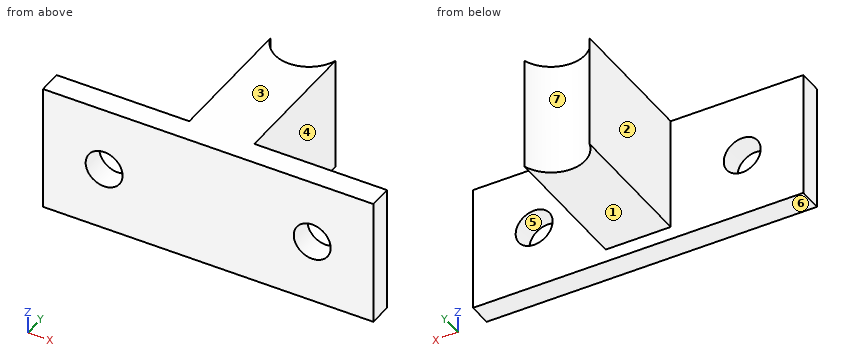
Autodesk Fusion 360 part; units mm, degrees
sketch "Sketch1" plane through (0, 0, 0) normal (0, 1, 0) x (1, 0, 0)
  line L0 (2.5, -4.375) -> (-2.5, -4.375)
  line L1 (-2.5, -4.375) -> (-2.5, 4.375)
  line L2 (-2.5, 4.375) -> (2.5, 4.375)
  line L3 (2.5, 4.375) -> (2.5, -4.375)
  line L4 (0, -17.6215) -> (0, 10.113) construction
  line L5 (14.6118, 0) -> (-14.9327, 0) construction
  dimension "d1" = 5
  dimension "d2" = 8.75
extrude "Extrude1" add sketch "Sketch1" along normal blind 8.875
sketch "Sketch2" plane through (0, 0, 4.375) normal (0, 0, 1) x (1, 0, 0)
  line L0 (-2.5, 0) -> (2.5, 0)
  line L1 (2.5, 0) -> (2.5, 8.875)
  line L2 (2.5, 8.875) -> (-2.5, 8.875)
  line L3 (-2.5, 8.875) -> (-2.5, 0)
  line L4 (-2.5, 8.875) -> (2.5, 8.875)
  line L5 (2.5, 8.875) -> (2.5, 11.5)
  line L6 (2.5, 11.5) -> (-2.5, 11.5)
  line L7 (-2.5, 11.5) -> (-2.5, 8.875)
  circle A0 centre (0, 11.5) radius 2.625
  line L8 (0, 0) -> (0, 8.875) construction
  dimension "d10" = 5.25
extrude "Extrude3" add sketch "Sketch2" against normal blind 8.75 contours L2 L4 L7 A0 | L2 L4 L5 A0
sketch "Sketch3" plane through (0, 0, 0) normal (0, -1, 0) x (1, 0, 0)
  line L0 (-2.5, -4.375) -> (2.5, -4.375)
  line L1 (2.5, -4.375) -> (2.5, 4.375)
  line L2 (2.5, 4.375) -> (-2.5, 4.375)
  line L3 (-2.5, 4.375) -> (-2.5, -4.375)
  line L4 (-12.7, 4.375) -> (12.7, 4.375)
  line L5 (12.7, 4.375) -> (12.7, -5.375)
  line L6 (12.7, -5.375) -> (-12.7, -5.375)
  line L7 (-12.7, -5.375) -> (-12.7, 4.375)
  line L8 (0, 4.375) -> (0, -4.375) construction
  line L9 (12.7, -0.5) -> (-12.7, -0.5) construction
  circle A0 centre (-8, -0.5) radius 1.42
  circle A1 centre (8, -0.5) radius 1.42
  dimension "d16" = 25.4
  dimension "d17" = 2.84
  dimension "d18" = 16
  dimension "d21" = 9.75
  dimension "d22" = 4.875
extrude "Extrude5" add sketch "Sketch3" along normal blind 1.8
The model under review builds one solid part; all positions refer to its coordinate system, in mm. Face numbers are marked on the shaded views. A direction names the side the tool comes from. Round coordinates to 2 decimals unless told otherwise and drop trailing zeros. Order: outer loops, then holes, each group sorted by start corner. A loop starts at its lowest first (then second) coordinate and runs counter-clockwise, first axis right, second up. Notation, with made-up numbers: (41.25, 49.25) - (68.25, 49.25) arc R11 ccw to (68.25, 66.25) - close; hole circle Ø3 at (80.5, -16). An arc over 180 degrees is marked (long way). Answer in a Markdown table with one row per item.
(1) For line 1 (Z direction, x = 8, y = -1.35) (3 decimals); line 2 (X direction, y = 9.75, z = 2.5); line 3 (Y direction, x = 4.75, z = -3.5), list the stretches that pass through material, from the lowest coordinate up. Write a range as from..to.
Result set:
| item | result |
|---|---|
| line 1 | z = -5.375..-1.92, 0.92..4.375 |
| line 2 | x = -2.5..-1.96, 1.96..2.5 |
| line 3 | y = -1.8..0 |
(2) Take a section at C-C on y = 10. Write out the cut boundary in (x, z) (3 decimals), plus the area to 3 significant figures.
Result set:
| item | result |
|---|---|
| outline | (-2.5, -4.375) - (-2.154, -4.375) - (-2.154, 4.375) - (-2.5, 4.375) - close; (2.154, -4.375) - (2.5, -4.375) - (2.5, 4.375) - (2.154, 4.375) - close |
| area | 6.05 mm2 |
(3) Machinability: for the marked faces 1, 2 and 3, which of the approach directions +Z, -Z, +X, -X, +Y, -Y give a long, thin tool a straight path to every point of the face, cutting with its end or side? Answer none if there is none.
Result set:
| item | result |
|---|---|
| face 1 | -Z, +X, -X, +Y |
| face 2 | +Z, -Z, -X, +Y |
| face 3 | +Z, +X, -X, +Y, -Y |
(4) Take a section at B-B on x = 8. Write out the cut boundary in (y, z) (3 decimals), plus the area to 3 significant figures.
Result set:
| item | result |
|---|---|
| outline | (-1.8, -5.375) - (0, -5.375) - (0, -1.92) - (-1.8, -1.92) - close; (-1.8, 0.92) - (0, 0.92) - (0, 4.375) - (-1.8, 4.375) - close |
| area | 12.4 mm2 |
(5) Take a section at D-D on x = 0. Write out the cut boundary in (y, z) (3 decimals).
Result set:
| item | result |
|---|---|
| outline | (-1.8, -5.375) - (0, -5.375) - (0, -4.375) - (8.875, -4.375) - (8.875, 4.375) - (-1.8, 4.375) - close |
(6) Take a section at A-A on z = -0.5. Write out the cut boundary in (x, y) (3 decimals), plus the area to 3 significant figures.
Result set:
| item | result |
|---|---|
| outline | (-12.7, -1.8) - (-9.42, -1.8) - (-9.42, 0) - (-12.7, 0) - close; (-6.58, -1.8) - (6.58, -1.8) - (6.58, 0) - (2.5, 0) - (2.5, 10.7) arc R2.625 cw to (-2.5, 10.7) - (-2.5, 0) - (-6.58, 0) - close; (9.42, -1.8) - (12.7, -1.8) - (12.7, 0) - (9.42, 0) - close |
| area | 82.3 mm2 |
(7) Mouldability with a two-part tool opening along X and no side actions: class the marked faces 4, 5, 6 and 7 as released by +X, released by -X, zero draft, split by the parting line, or undercut.
Result set:
| item | result |
|---|---|
| face 4 | released by +X |
| face 5 | undercut |
| face 6 | zero draft |
| face 7 | undercut |
(8) Clearance check with flat-ended pins moving along their axes: P1, Ø5, axis at y = 1, z = -3.5, coming from the -X side; P2, Ø5.5, axis at x = 0, y = 4.5, coming from the -Z side (3 decimals); P3, Ø4.5, axis at x = -8, z = -0.5, coming from the +Y side. State where each tip first meets the part, or that it passes through.
Result set:
| item | result |
|---|---|
| P1 | stops at x = -12.7 |
| P2 | stops at z = -4.375 |
| P3 | stops at y = 0 |
